Geometry check sheet. Reference: the model listing, model coordinates, mm. A direction names the side the tool comes from. Coordinates: 2 decimals unless noted, no trailing zeros. Write each loop counter-clockwise with the first axis right and the second up, starting at its lowest first coordinate (ties: lowest second). Pieces come first, ordered by that corner, then holes. Notation, with made-up numbers: (43.25, 47) -> (50.25, 47) arc R16 ccw to (50.25, 61) -> close; hole circle Ø1 at (81.25, 6). An arc over 180 degrees is marked (long way). Use a Markdown table: item, result.
```python
from build123d import *

# Parameters (mm, degrees)
SKETCH2_R           = 1.75
BOSS_EXTRUDE2_DEPTH = 27
SKETCH3_R           = 1.75
SKETCH3_W           = 8.65
SKETCH3_H           = 7
CUT_EXTRUDE1_DEPTH  = 30
SKETCH4_R           = 3
CUT_EXTRUDE2_DEPTH  = 3


with BuildPart() as part:
    # Sketch2 → Boss-Extrude2 (new body)
    with BuildSketch(Plane(origin=(0, 0, 0), x_dir=(0, 0, -1), z_dir=(1, 0, 0))):
        with BuildLine():
            Line((0, -3), (17, -3))
            Line((17, -3), (17, 3))
            Line((17, 3), (0, 3))
            ThreePointArc((0, 3), (-3, 0), (0, -3))
        make_face()
        Circle(SKETCH2_R, mode=Mode.SUBTRACT)
    extrude(amount=BOSS_EXTRUDE2_DEPTH)

    # Sketch3 → Cut-Extrude1 (cut)
    with BuildSketch(Plane.XZ.offset(3)):
        with Locations((3.5, -11.5)):
            Circle(SKETCH3_R)
        with Locations((23.5, -11.5)):
            Circle(SKETCH3_R)
        with Locations((22.675, -0.5)):
            Rectangle(SKETCH3_W, SKETCH3_H)
        with Locations((4.325, -0.5)):
            Rectangle(SKETCH3_W, SKETCH3_H)
    extrude(amount=-CUT_EXTRUDE1_DEPTH, mode=Mode.SUBTRACT)

    # Sketch4 → Cut-Extrude2 (cut)
    with BuildSketch(Plane.XZ.offset(3)):
        with Locations((3.5, -11.5)):
            Circle(SKETCH4_R)
        with Locations((23.5, -11.5)):
            Circle(SKETCH4_R)
    extrude(amount=-CUT_EXTRUDE2_DEPTH, mode=Mode.SUBTRACT)


solid = part.part
```
Item 1: Section check C-C on y = 1.35. Record the boundary of the cut face in (x, z), then the cut area to 3 significant figures.
Answer block:
| item | result |
|---|---|
| outline | (0, -17) -> (27, -17) -> (27, -4) -> (18.35, -4) -> (18.35, -1.11) -> (8.65, -1.11) -> (8.65, -4) -> (0, -4) -> close; (8.65, 1.11) -> (18.35, 1.11) -> (18.35, 2.68) -> (8.65, 2.68) -> close; hole circle Ø3.5 at (3.5, -11.5); hole circle Ø3.5 at (23.5, -11.5) |
| area | 375 mm^2 |
Item 2: Thickness scan on L1, parallel to X at y = -1.8, z = -13.75; L2, parallel to Z at x = 3.5, y = -1.1; L3, parallel to Z at x = 23.5, y = 2.35. Record the ranges inside material, lowest first. Write a range as [from, to].
Answer block:
| item | result |
|---|---|
| L1 | x = [0, 1.52], [5.48, 21.52], [25.48, 27] |
| L2 | z = [-17, -14.5], [-8.5, -4] |
| L3 | z = [-17, -13.25], [-9.75, -4] |
Item 3: Tool access check on faces 4 (the flat face through (23, 0, -4)), 5 (the flat face through (4, 0, -4)), 6 (the cylindrical face through (0.5, -1.5, -11.4)). Record the directions out of +Z, -Z, +X, -X, +Y, -Y that give a thin tool (end or side, any length) a straight path to the whole face; none if there is none.
Answer block:
| item | result |
|---|---|
| face 4 | +Z, +X, +Y, -Y |
| face 5 | +Z, -X, +Y, -Y |
| face 6 | -Y |
Item 4: Section check D-D on y = -2.05. Record the boundary of the cut face in (x, z).
Answer block:
| item | result |
|---|---|
| outline | (0, -17) -> (27, -17) -> (27, -4) -> (18.35, -4) -> (18.35, 2.19) -> (8.65, 2.19) -> (8.65, -4) -> (0, -4) -> close; hole circle Ø6 at (3.5, -11.5); hole circle Ø6 at (23.5, -11.5) |
Item 5: Section check B-B on x = 24.75. Record the boundary of the cut face in (y, z).
Answer block:
| item | result |
|---|---|
| outline | (-3, -17) -> (3, -17) -> (3, -12.72) -> (0, -12.72) -> (0, -14.23) -> (-3, -14.23) -> close; (-3, -8.77) -> (0, -8.77) -> (0, -10.28) -> (3, -10.28) -> (3, -4) -> (-3, -4) -> close |
Item 6: Mould release check, pull along X, two halves, no side actions. Record for faces 1 (the flat face through (27, 0, -10)), 2 (the cylindrical face through (20.5, -1.5, -11.4)), 3 (the flat face through (8.65, 0, -2)): +X half, -X half, draft (parallel to the pull), parting line (faces both ways), or undercut.
Answer block:
| item | result |
|---|---|
| face 1 | +X half |
| face 2 | undercut |
| face 3 | -X half |
Item 7: Section check A-A on z = -11.5. Record the boundary of the cut face in (x, y).
Answer block:
| item | result |
|---|---|
| outline | (0, -3) -> (0.5, -3) -> (0.5, 0) -> (1.75, 0) -> (1.75, 3) -> (0, 3) -> close; (5.25, 0) -> (6.5, 0) -> (6.5, -3) -> (20.5, -3) -> (20.5, 0) -> (21.75, 0) -> (21.75, 3) -> (5.25, 3) -> close; (25.25, 0) -> (26.5, 0) -> (26.5, -3) -> (27, -3) -> (27, 3) -> (25.25, 3) -> close |
Item 8: Depth check by flat-ended pin: P1, Ø4, axis at x = 3.5, z = -11.5, coming from the -Y side; P2, Ø1.8, axis at y = -0.5, z = -1, coming from the -X side. Enter the tip coordinate at first touch or a pass-through.
Answer block:
| item | result |
|---|---|
| P1 | stops at y = 0 |
| P2 | stops at x = 8.65 |
